Read the model definition and answer for the solid it produces. Units are mm, in the model's axes. Face numbers are marked on the shaded views. A direction names the side the tool comes from. Give positions to 0.01 mm unless a question says otherwise; leave off trailing zeros. Order: outer loops, then holes, each group sorted by start corner. A loop starts at its lowest first (then second) coordinate and runs counter-clockwise, first axis right, second up.
```python
from build123d import *

# Parameters (mm, degrees)
SKETCH1_W           = 160
SKETCH1_H           = 50
BOSS_EXTRUDE1_DEPTH = 8
SKETCH2_W           = 10
SKETCH2_H           = 50
BOSS_EXTRUDE2_DEPTH = 50
SKETCH3_W           = 9.9
SKETCH3_H           = 29.9
BOSS_EXTRUDE3_DEPTH = 10
CUT_EXTRUDE1_REACH  = 70
SKETCH4_R           = 2.15


with BuildPart() as part:
    # Sketch1 → Boss-Extrude1 (new body)
    with BuildSketch(Plane(origin=(0, 0, 0), x_dir=(1, 0, 0), z_dir=(0, 1, 0))):
        Rectangle(SKETCH1_W, SKETCH1_H)
    extrude(amount=BOSS_EXTRUDE1_DEPTH)

    # Sketch2 → Boss-Extrude2 (add)
    with BuildSketch(Plane(origin=(0, 8, 0), x_dir=(1, 0, 0), z_dir=(0, 1, 0))):
        with Locations((-75, 0)):
            Rectangle(SKETCH2_W, SKETCH2_H)
        with Locations((75, 0)):
            Rectangle(SKETCH2_W, SKETCH2_H)
    extrude(amount=BOSS_EXTRUDE2_DEPTH)

    # Sketch3 → Boss-Extrude3 (add)
    with BuildSketch(Plane(origin=(0, 58, 0), x_dir=(1, 0, 0), z_dir=(0, 1, 0))):
        with Locations((-75, 0)):
            Rectangle(SKETCH3_W, SKETCH3_H)
        with Locations((75, 0)):
            Rectangle(SKETCH3_W, SKETCH3_H)
    extrude(amount=BOSS_EXTRUDE3_DEPTH)

    # Sketch4 → Cut-Extrude1 (cut, up to next)
    with BuildSketch(Plane.XZ, mode=Mode.PRIVATE) as cut_extrude1_sk1:
        Circle(SKETCH4_R)
    cut_extrude1_tool1 = extrude(cut_extrude1_sk1.sketch, amount=-CUT_EXTRUDE1_REACH, mode=Mode.PRIVATE) & part.part
    add(cut_extrude1_tool1.solids().sort_by_distance((0, 0, 0))[0], mode=Mode.SUBTRACT)
    # Sketch4 → Cut-Extrude1 (cut, up to next)
    with BuildSketch(Plane.XZ, mode=Mode.PRIVATE) as cut_extrude1_sk2:
        with Locations((-11.313708499, 11.313708499)):
            Circle(SKETCH4_R)
    cut_extrude1_tool2 = extrude(cut_extrude1_sk2.sketch, amount=-CUT_EXTRUDE1_REACH, mode=Mode.PRIVATE) & part.part
    add(cut_extrude1_tool2.solids().sort_by_distance((-11.313708, 0, 11.313708))[0], mode=Mode.SUBTRACT)
    # Sketch4 → Cut-Extrude1 (cut, up to next)
    with BuildSketch(Plane.XZ, mode=Mode.PRIVATE) as cut_extrude1_sk3:
        with Locations((11.313708499, 11.313708499)):
            Circle(SKETCH4_R)
    cut_extrude1_tool3 = extrude(cut_extrude1_sk3.sketch, amount=-CUT_EXTRUDE1_REACH, mode=Mode.PRIVATE) & part.part
    add(cut_extrude1_tool3.solids().sort_by_distance((11.313708, 0, 11.313708))[0], mode=Mode.SUBTRACT)
    # Sketch4 → Cut-Extrude1 (cut, up to next)
    with BuildSketch(Plane.XZ, mode=Mode.PRIVATE) as cut_extrude1_sk4:
        with Locations((11.313708499, -11.313708499)):
            Circle(SKETCH4_R)
    cut_extrude1_tool4 = extrude(cut_extrude1_sk4.sketch, amount=-CUT_EXTRUDE1_REACH, mode=Mode.PRIVATE) & part.part
    add(cut_extrude1_tool4.solids().sort_by_distance((11.313708, 0, -11.313708))[0], mode=Mode.SUBTRACT)
    # Sketch4 → Cut-Extrude1 (cut, up to next)
    with BuildSketch(Plane.XZ, mode=Mode.PRIVATE) as cut_extrude1_sk5:
        with Locations((-11.313708499, -11.313708499)):
            Circle(SKETCH4_R)
    cut_extrude1_tool5 = extrude(cut_extrude1_sk5.sketch, amount=-CUT_EXTRUDE1_REACH, mode=Mode.PRIVATE) & part.part
    add(cut_extrude1_tool5.solids().sort_by_distance((-11.313708, 0, -11.313708))[0], mode=Mode.SUBTRACT)


solid = part.part
```
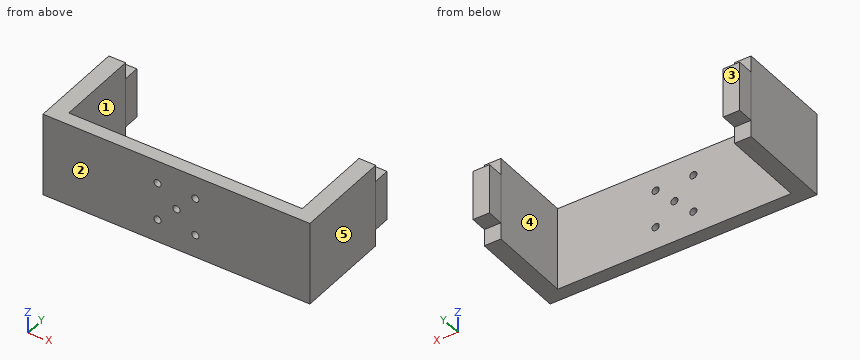
1) The part is cut by section A-A on z = 0. Determine the outline of the cut face in (x, y).
Final values:
outline: (-80, 0) - (-2.15, 0) - (-2.15, 8) - (-70, 8) - (-70, 58) - (-70.05, 58) - (-70.05, 68) - (-79.95, 68) - (-79.95, 58) - (-80, 58) - close; (2.15, 0) - (80, 0) - (80, 58) - (79.95, 58) - (79.95, 68) - (70.05, 68) - (70.05, 58) - (70, 58) - (70, 8) - (2.15, 8) - close
2) Given pin 1 (3.5 mm diameter, centred on x = -11.31, z = 11.31, fed in from +Y); pin 2 (12 mm diameter, centred on x = -33.5, z = -12.5, fed in from +Y); pin 3 (5 mm diameter, centred on x = 73.5, y = 62, fed in from -Z); pin 4 (3 mm diameter, centred on x = -73.5, y = 63.5, fed in from +Z), each flat-ended and moving along its own axis, determine where each tip first touches the part or whether it passes through.
Final values:
pin 1: passes through
pin 2: stops at y = 8
pin 3: stops at z = -14.95
pin 4: stops at z = 14.95
3) The part is cut by section C-C on x = 0. Determine the outline of the cut face in (y, z), and give its area (3 significant figures).
Final values:
outline: (0, -25) - (8, -25) - (8, -2.15) - (0, -2.15) - close; (0, 2.15) - (8, 2.15) - (8, 25) - (0, 25) - close
area: 366 mm2
4) The part is cut by section D-D on x = 59. Determine the outline of the cut face in (y, z).
Final values:
outline: (0, -25) - (8, -25) - (8, 25) - (0, 25) - close
5) For a pull along X with two mould halves and no side action, classify the marked faces 3, 4 and 5 as released by +X, released by -X, zero draft, split by the parting line, or undercut.
Final values:
face 3: zero draft
face 4: undercut
face 5: released by +X
6) Consider L1, parallel to Z at x = 0, y = 5; L2, parallel to X at y = 46, z = 3; L3, parallel to Y at x = 35, z = 19. Determine where each line is inside the solid, lowest interval first.
Final values:
L1: z = -25 to -2.15, 2.15 to 25
L2: x = -80 to -70, 70 to 80
L3: y = 0 to 8
7) The part is cut by section B-B on y = 44. Determine the outline of the cut face in (x, z).
Final values:
outline: (-80, -25) - (-70, -25) - (-70, 25) - (-80, 25) - close; (70, -25) - (80, -25) - (80, 25) - (70, 25) - close
8) A tool of negligible diameter and unlimited length cuts with its end or side. For the marked faces 1 and 2, from which of +Z, -Z, +X, -X, +Y, -Y can it reach the whole face along a straight path? Write none if from no direction.
Final values:
face 1: +Z, -Z, +Y
face 2: +Z, -Z, +X, -X, -Y
